Verification items for the finished model (mm, model axes). A direction names the side the tool comes from. Coordinates: 2 decimals unless noted, no trailing zeros. Order: outer loops, then holes, each group sorted by start corner. A loop starts at its lowest first (then second) coordinate and runs counter-clockwise, first axis right, second up. Notation, with made-up numbers: M -10,0.5 L 6,0.5 A26 cw 6,34.5 Z; hole C -20.75,-7.75 d4. An arc over 180 degrees is marked long. Return JSON: item names as keys, results as strings.
```python
from build123d import *

# Parameters (mm, degrees)
BOSS_EXTRUDE1_DEPTH = 28
SKETCH3_R           = 12.5
BOSS_EXTRUDE2_DEPTH = 5


with BuildPart() as part:
    # Sketch1 → Boss-Extrude1 (new body)
    with BuildSketch(Plane.XY):
        Polygon((5.85, 0), (5.85, -5.5), (-5.85, -5.5), (-5.85, 0), (-10.95, 0), (-10.95, 6.9), (10.95, 6.9), (10.95, 0), align=None)
    extrude(amount=-BOSS_EXTRUDE1_DEPTH)

    # Sketch3 → Boss-Extrude2 (add)
    with BuildSketch(Plane.XZ.offset(5.5)):
        with Locations(Location((0, -14, 0), (0, 0, 62.095449663))):
            Circle(SKETCH3_R)
    extrude(amount=BOSS_EXTRUDE2_DEPTH)


solid = part.part
```
Q1. Draft check along Z on faces 5 (the face through (-8, -5.5, -13)), 6 (the face through (0, 2, -28)), 7 (the face through (0, 2, 0)), 8 (the face through (2.079, -7.965, -26.326)). Enter one of: pulls with the +Z half, pulls with the -Z half, needs draft (parallel to the pull), parting line crosses it, or undercut.
Values:
{"face 5": "needs draft", "face 6": "pulls with the -Z half", "face 7": "pulls with the +Z half", "face 8": "parting line crosses it"}
Q2. Cross-section at B-B, the plane z = -14. Record the boundary of the cut face in (x, y), and give its area (3 significant figures).
Values:
{"outline": "M -12.5,-10.5 L 12.5,-10.5 L 12.5,-5.5 L 5.85,-5.5 L 5.85,0 L 10.95,0 L 10.95,6.9 L -10.95,6.9 L -10.95,0 L -5.85,0 L -5.85,-5.5 L -12.5,-5.5 Z", "area": "340 mm^2"}
Q3. Cross-section at C-C, the plane y = -4.5. Record the boundary of the cut face in (x, z).
Values:
{"outline": "M -5.85,-28 L 5.85,-28 L 5.85,0 L -5.85,0 Z"}
Q4. Material ranges on line 1 along Y through (x, z) = (7.5, -10.25); line 2 along X through (y, z) = (1.5, -25.25); line 3 along X through (y, z) = (-0.5, -6.75), recorded low to high.
Values:
{"line 1": "-10.5 to -5.5, 0 to 6.9", "line 2": "-10.95 to 10.95", "line 3": "-5.85 to 5.85"}
Q5. Tool access check on faces 1 (the face through (9, -5.5, -13)), 2 (the face through (10.95, 3, -14)), 3 (the face through (-8, 0, -14)), 4 (the face through (-10.95, 3, -14)). Record the directions out of +Z, -Z, +X, -X, +Y, -Y that give a thin tool (end or side, any length) a straight path to the whole face; none if there is none.
Values:
{"face 1": "+Z, -Z, +X", "face 2": "+Z, -Z, +X, +Y", "face 3": "+Z, -Z, -X", "face 4": "+Z, -Z, -X, +Y"}
Q6. Go/stop test with flat-tipped pins: pin 1 (1 mm diameter, centred on y = 1, z = -25, fed in from +X); pin 2 (3 mm diameter, centred on x = 2, y = -7.5, fed in from -Z); pin 3 (8 mm diameter, centred on y = -5, z = -19, fed in from -X). Record where each tip stops, or that it passes through.
Values:
{"pin 1": "x = 10.95", "pin 2": "z = -26.49", "pin 3": "x = -12.46"}
Q7. Cross-section at D-D, the plane x = 3.5. Record the boundary of the cut face in (y, z).
Values:
{"outline": "M -10.5,-26 L -5.5,-26 L -5.5,-28 L 6.9,-28 L 6.9,0 L -5.5,0 L -5.5,-2 L -10.5,-2 Z"}
Q8. Cross-section at A-A, the plane x = 0. Record the boundary of the cut face in (y, z), and give its area (3 significant figures).
Values:
{"outline": "M -10.5,-26.5 L -5.5,-26.5 L -5.5,-28 L 6.9,-28 L 6.9,0 L -5.5,0 L -5.5,-1.5 L -10.5,-1.5 Z", "area": "472 mm^2"}
